from build123d import *

# Parameters (mm, degrees)
SKETCH1_R           = 1
SKETCH1_R_2         = 2.5
BOSS_EXTRUDE1_DEPTH = 2
SKETCH2_R           = 3.65
SKETCH2_R_2         = 2.5
BOSS_EXTRUDE2_DEPTH = 2.5


with BuildPart() as part:
    # Sketch1 → Boss-Extrude1 (new body)
    with BuildSketch(Plane(origin=(0, 0, 0), x_dir=(1, 0, 0), z_dir=(0, 1, 0))):
        with BuildLine():
            Line((3, -2.079062289), (1.993477511, -14.51139211))
            ThreePointArc((1.993477511, -14.51139211), (0, -16.35), (-1.993477511, -14.51139211))
            Line((-1.993477511, -14.51139211), (-3, -2.079062289))
            ThreePointArc((-3, -2.079062289), (0, 3.65), (3, -2.079062289))
        make_face()
        with Locations((0, -6.65)):
            Circle(SKETCH1_R, mode=Mode.SUBTRACT)
        with Locations((0, -10.65)):
            Circle(SKETCH1_R, mode=Mode.SUBTRACT)
        Circle(SKETCH1_R_2, mode=Mode.SUBTRACT)
    extrude(amount=BOSS_EXTRUDE1_DEPTH)

    # Sketch2 → Boss-Extrude2 (add)
    with BuildSketch(Plane(origin=(0, 2, 0), x_dir=(1, 0, 0), z_dir=(0, 1, 0))):
        Circle(SKETCH2_R)
        Circle(SKETCH2_R_2, mode=Mode.SUBTRACT)
    extrude(amount=BOSS_EXTRUDE2_DEPTH)


solid = part.part
The listing builds one solid part. Answer for the finished solid, in the listing's coordinates (mm). Coordinates: 2 decimals unless noted, no trailing zeros. Loops run counter-clockwise (first coordinate to the right, second up) from the corner with the lowest first, then second, coordinate; pieces in that order, holes last.
1) Find section B-B on z = 0. Write down the section's boundary in (x, y), then the cut area to 4 significant figures.
2) Find the intervals of material crossed by L1, parallel to X at y = 3.3, z = 0; L2, parallel to Z at x = -0.75, y = 0.35, in increasing order.
3) Find section A-A on x = 0. Write down the section's boundary in (y, z).
4) A flat-ended cylindrical pin translates along its axis: pin 1 Ø2.5 at (x, z) = (0, 10.65) entering from +Y. Find the tip coordinate at first contact, or state that the pin passes through.
5) Find section C-C on y = 0.4. Write down the section's boundary in (x, z), then the cut area to 3 significant figures.
6) Find section D-D on y = 4. Write down the section's boundary in (x, z).
7) Determine the mould class of faces 1 (the face through (0, 2, 9)), 2 (the face through (-0.54, 2.22, 2.44)), 3 (the face through (2.504, 0.986, 8.208)) for opening direction Z: pulls with the +Z half, pulls with the -Z half, needs draft (parallel to the pull), parting line crosses it, or undercut.
Values:
1. outline: (-3.65, 0) - (-2.5, 0) - (-2.5, 4.5) - (-3.65, 4.5) - close; (2.5, 0) - (3.65, 0) - (3.65, 4.5) - (2.5, 4.5) - close
1. area: 10.35 mm2
2. L1: x = -3.65 to -2.5, 2.5 to 3.65
2. L2: z = -3.57 to -2.38, 2.38 to 5.99, 7.31 to 9.99, 11.31 to 16.2
3. outline: (0, -3.65) - (4.5, -3.65) - (4.5, -2.5) - (0, -2.5) - close; (0, 2.5) - (4.5, 2.5) - (4.5, 3.65) - (2, 3.65) - (2, 5.65) - (0, 5.65) - close; (0, 7.65) - (2, 7.65) - (2, 9.65) - (0, 9.65) - close; (0, 11.65) - (2, 11.65) - (2, 16.35) - (0, 16.35) - close
4. pin 1: stops at y = 2
5. outline: (-3, 2.08) arc R3.65 ccw (long way) to (3, 2.08) - (1.99, 14.51) arc R2 ccw to (-1.99, 14.51) - close; hole circle Ø5 at (0, 0); hole circle Ø2 at (0, 6.65); hole circle Ø2 at (0, 10.65)
5. area: 77.0 mm2
6. outline: circle Ø7.3 at (0, 0); hole circle Ø5 at (0, 0)
7. face 1: needs draft
7. face 2: undercut
7. face 3: pulls with the +Z half
